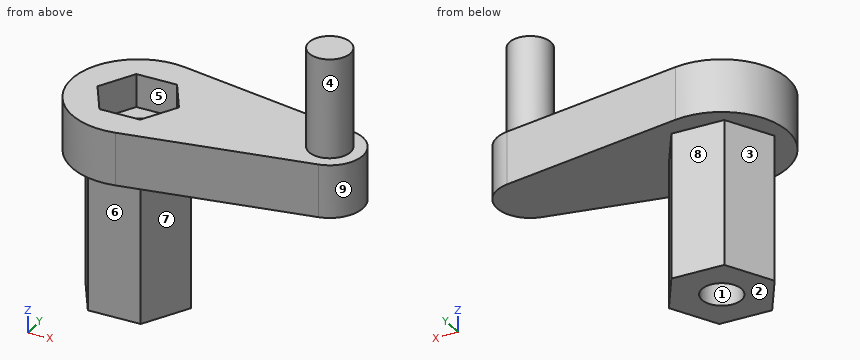
from build123d import *

# Parameters (mm, degrees)
PAD046_DEPTH    = 22
PAD047_DEPTH    = 8
SKETCH080_R     = 3.125
PAD048_DEPTH    = 15
SKETCH081_R     = 3
HOLE_DEPTH      = 30.001
POCKET037_DEPTH = 5


with BuildPart() as part:
    # Sketch078 → Pad046 (new body)
    with BuildSketch(Plane.XY):
        Polygon((3.933199, 6.8125), (-3.933199, 6.8125), (-7.866397, 0), (-3.933199, -6.8125), (3.933199, -6.8125), (7.866397, 0), align=None)
    extrude(amount=PAD046_DEPTH)

    # Sketch079 (on Face8 of Pad046) → Pad047 (join)
    with BuildSketch(Plane.XY.offset(22)):
        with BuildLine():
            ThreePointArc((1.754386, 9.844904), (-10, 0), (1.754386, -9.844904))
            Line((1.754386, -9.844904), (29.377193, -4.922452))
            ThreePointArc((29.377193, -4.922452), (33.5, 0), (29.377193, 4.922452))
            Line((29.377193, 4.922452), (1.754386, 9.844904))
        make_face()
    extrude(amount=PAD047_DEPTH)

    # Sketch080 (on Face5 of Pad047) → Pad048 (join)
    with BuildSketch(Plane.XY.offset(30)):
        with Locations((28.5, 0)):
            Circle(SKETCH080_R)
    extrude(amount=PAD048_DEPTH)

    # Sketch081 (on Face5 of Pad048) → Hole (cut, through all)
    with BuildSketch(Plane.XY.offset(30)):
        Circle(SKETCH081_R)
    extrude(amount=-HOLE_DEPTH, mode=Mode.SUBTRACT)

    # Sketch082 (on Face5 of Hole) → Pocket037 (cut)
    with BuildSketch(Plane.XY.offset(30)):
        Polygon((3.031089, 5.25), (-3.031089, 5.25), (-6.062178, 0), (-3.031089, -5.25), (3.031089, -5.25), (6.062178, 0), align=None)
    extrude(amount=-POCKET037_DEPTH, mode=Mode.SUBTRACT)


solid = part.part
Design review of the part built by this model. Coordinates are the model's own, in mm. Face numbers are marked on the shaded views. A direction names the side the tool comes from. Give positions to 0.01 mm unless a question says otherwise; leave off trailing zeros. Order: outer loops, then holes, each group sorted by start corner. A loop starts at its lowest first (then second) coordinate and runs counter-clockwise, first axis right, second up. Notation, with made-up numbers: (-11.5, 49.25) - (-1.5, 49.25) arc R17 cw to (-1.5, 59.25) - close; hole circle Ø7 at (37.25, 85.25). An arc over 180 degrees is marked (long way). Write item = value, one per line. Start each with the question number.
Q1. We need section A-A on z = 26. State the section outline as (x, y) points.
Q2. To check wall thickness, follow L1, parallel to Y at x = 0, z = 18.25; L2, parallel to X at y = 0, z = 29.5; L3, parallel to Y at x = -3.5, z = 20.5. State the ranges of each line that lie inside material, in increasing order. Write a range as from..to.
Q3. We need section C-C on y = -2. State the section outline as (x, z) points, plus the area to 3 significant figures.
Q4. Clearance check with flat-ended pins moving along their axes: pin 1 Ø4 at (x, z) = (-1, 12.5) entering from +Y; pin 2 Ø1.5 at (y, z) = (6, 30) entering from -X; pin 3 Ø2.5 at (x, z) = (-1.5, 11) entering from -Y; pin 4 Ø5 at (x, y) = (0, 0) entering from -Z. State where each tip first meets the part, or that it passes through.
Q5. Mouldability with a two-part tool opening along X and no side actions: class the marked faces 1, 2, 3 and 4 as released by +X, released by -X, zero draft, split by the parting line, or undercut.
Q6. We need section D-D on x = -4.5. State the section outline as (y, z) points.
Q7. Tool access review of the marked faces 5, 6, 7, 8 and 9: name each direction out of +Z, -Z, +X, -X, +Y, -Y from which nothing blocks a thin tool from reaching the whole face with its end or side.
Q8. We need section B-B on x = 0. State the section outline as (y, z) points.
Working result:
q1.outline = (1.75, -9.84) - (29.38, -4.92) arc R5 ccw to (29.38, 4.92) - (1.75, 9.84) arc R10 ccw (long way) to start; hole (-6.06, 0) - (-3.03, -5.25) - (3.03, -5.25) - (6.06, 0) - (3.03, 5.25) - (-3.03, 5.25) - close
q2.L1 = -6.81..-3, 3..6.81
q2.L2 = -10..-6.06, 6.06..33.5
q2.L3 = -6.81..6.81
q3.outline = (-9.8, 22) - (-6.71, 22) - (-6.71, 0) - (-2.24, 0) - (-2.24, 25) - (-4.91, 25) - (-4.91, 30) - (-9.8, 30) - close; (2.24, 0) - (6.71, 0) - (6.71, 22) - (33.08, 22) - (33.08, 30) - (30.9, 30) - (30.9, 45) - (26.1, 45) - (26.1, 30) - (4.91, 30) - (4.91, 25) - (2.24, 25) - close
q3.area = 550 mm²
q4.pin_1 = 6.81
q4.pin_2 = -8.51
q4.pin_3 = -6.81
q4.pin_4 = through
q5.face_1 = undercut
q5.face_2 = zero draft
q5.face_3 = released by -X
q5.face_4 = split by the parting line
q6.outline = (-8.93, 22) - (-5.83, 22) - (-5.83, 0) - (5.83, 0) - (5.83, 22) - (8.93, 22) - (8.93, 30) - (2.71, 30) - (2.71, 25) - (-2.71, 25) - (-2.71, 30) - (-8.93, 30) - close
q7.face_5 = +Z
q7.face_6 = -Z, +X, -X, -Y
q7.face_7 = -Z, +X, -Y
q7.face_8 = -Z, +X, -X, +Y
q7.face_9 = +Z, -Z, +X
q8.outline = (-10, 22) - (-6.81, 22) - (-6.81, 0) - (-3, 0) - (-3, 25) - (-5.25, 25) - (-5.25, 30) - (-10, 30) - close; (3, 0) - (6.81, 0) - (6.81, 22) - (10, 22) - (10, 30) - (5.25, 30) - (5.25, 25) - (3, 25) - close
